The model under review builds one solid part; all positions refer to its coordinate system, in mm. A direction names the side the tool comes from. Round coordinates to 2 decimals unless told otherwise and drop trailing zeros. Order: outer loops, then holes, each group sorted by start corner. A loop starts at its lowest first (then second) coordinate and runs counter-clockwise, first axis right, second up.
1) Consider section A-A (y = 50). Give the boundary of the cut face in (x, z), then the cut area to 3 significant figures.
2) Consider section B-B (x = -3). Give the number of separate pieces and of enclosed holes in the cut face, then the cut area to 3 significant figures.
3) Clearance check with flat-ended pins moving along their axes: P1, Ø10.5, axis at x = -18, y = 14.5, coming from the -Z side; P2, Ø1.6, axis at x = -12.5, z = -1, coming from the +Y side; P3, Ø2.5, axis at x = -20, z = 3.5, coming from the +Y side; P4, Ø2.5, axis at x = 0, y = 59.563, coming from the -Z side. State where each tip first meets the part, or that it passes through.
4) Machinability: for faces 5 (the face through (-12, 0, -2)), 6 (the face through (12.29, 102.343, 3.073)), 7 (the face through (0, 0, 2)), which of the approach directions +Z, -Z, +X, -X, +Y, -Y give a long, thin tool a straight path to every point of the face, cutting with its end or side? Answer none if there is none.
5) Mouldability with a two-part tool opening along Y and no side actions: class faces 1 (the face through (-47.955, -39, 1)), 2 (the face through (-25.182, -23.28, -1.032)), 3 (the face through (17, 86.36, 2)), 4 (the face through (-0.05, 79.4, 2.44)) as pulls with the +Y half, pulls with the -Y half, needs draft (parallel to the pull), parting line crosses it, or undercut.
6) To check wall thickness, follow L1, parallel to Y at x = 1, z = 3.5; L2, parallel to Y at x = -21, z = -0.75; L3, parallel to Y at x = -8, z = 4.75. State the ranges of each line that lie inside material, in increasing order.
7) Consider section D-D (y = 93). Give the boundary of the cut face in (x, z), then the cut area to 3 significant figures.
from build123d import *

# Parameters (mm, degrees)
F1_DEPTH       = 4.953
F3_DEPTH       = 4.954
F5_DEPTH       = 109.983
F7_DEPTH       = 15.494
F8_W           = 74.6252
F8_H           = 44.45
F9_DEPTH       = 4.953
F9_DEPTH_BACK  = 3.175
F11_R          = 1.27
F17_DEPTH      = 3.176
F17_DEPTH_BACK = 4.954
F19_D          = 3.15
F20_R          = 3.302
F21_R          = 2.5393938838
F22_SIZE       = 2.286


# Not quite as in the source:
# - a feature names something its author has since deleted; it is built from what else it names


with BuildPart() as f1:
    # F0 (on Top) → F1 (new body)
    with BuildSketch(Plane.XY):
        Polygon((-26.67, 0), (26.67, 0), (26.67, 90.043), (16.9418, 109.982), (-16.9418, 109.982), (-26.67, 90.043), align=None)
    extrude(amount=F1_DEPTH)

    # F2 (on Top) → F3 (cut, through all)
    with BuildSketch(Plane.XY):
        with BuildLine():
            Line((-26.67, 28.0162), (-7.0612, 28.0162))
            ThreePointArc((-7.0612, 28.0162), (0.0508, 35.1282), (-7.0612, 42.2402))
            Line((-7.0612, 42.2402), (-26.67, 42.2402))
            Line((-26.67, 42.2402), (-26.67, 28.0162))
        make_face()
        with BuildLine():
            Line((26.67, 86.36), (7.0612, 86.36))
            ThreePointArc((7.0612, 86.36), (-0.0508, 79.248), (7.0612, 72.136))
            Line((7.0612, 72.136), (26.67, 72.136))
            Line((26.67, 72.136), (26.67, 86.36))
        make_face()
    extrude(amount=F3_DEPTH, mode=Mode.SUBTRACT)

    # F4 (on face) → F5 (cut, through all)
    with BuildSketch(Plane.XZ):
        with BuildLine():
            ThreePointArc((-11.0871, 0), (-12.3571, 1.27), (-13.6271, 0))
            Line((-13.6271, 0), (-11.0871, 0))
        make_face()
        with BuildLine():
            ThreePointArc((13.6271, 0), (12.3571, 1.27), (11.0871, 0))
            Line((11.0871, 0), (13.6271, 0))
        make_face()
    extrude(amount=-F5_DEPTH, mode=Mode.SUBTRACT)

    # F6 (on face) → F7 (cut)
    with BuildSketch(Plane(origin=(0, 109.982, 0), x_dir=(-1, 0, 0), z_dir=(0, 1, 0))):
        with BuildLine():
            ThreePointArc((-9.2837, 0), (-12.3571, 3.0734), (-15.4305, 0))
            Line((-15.4305, 0), (-9.2837, 0))
        make_face()
        with BuildLine():
            ThreePointArc((15.4305, 0), (12.3571, 3.0734), (9.2837, 0))
            Line((9.2837, 0), (15.4305, 0))
        make_face()
    extrude(amount=-F7_DEPTH, mode=Mode.SUBTRACT)

    # F8 (on Top) → F9 (join, two sides)
    with BuildSketch(Plane.XY) as f9_sk:
        with Locations((-10.6426, -22.225)):
            Rectangle(F8_W, F8_H)
    extrude(amount=F9_DEPTH)
    extrude(f9_sk.sketch, amount=-F9_DEPTH_BACK)

    # F12: sweep along a path in F10
    with BuildLine(Plane.XY) as f12_path:
        Line((-47.9552, -41.275), (-28.9179, -41.275))
        ThreePointArc((-28.9179, -41.275), (0.2679323935, -29.1858323935), (12.3571, 0))
    # F11 (on face) → F12 (sweep, cut)
    with BuildSketch(Plane(origin=(0, 0, 0), x_dir=(-1, 0, 0), z_dir=(0, 1, 0))):
        with Locations((-12.3571, 0)):
            Circle(F11_R)
    sweep(path=f12_path.line, mode=Mode.SUBTRACT)

    # F15: sweep along a path in F13
    with BuildLine(Plane.XY) as f15_path:
        ThreePointArc((-12.3571, 0), (-22.7835420926, -25.1716579074), (-47.9552, -35.5981))
    # F14 (on face) → F15 (sweep, cut)
    with BuildSketch(Plane(origin=(0, 0, 0), x_dir=(-1, 0, 0), z_dir=(0, 1, 0))):
        with BuildLine():
            ThreePointArc((11.0871, 0), (12.3571, -1.27), (13.6271, 0))
            ThreePointArc((13.6271, 0), (12.3571, 1.27), (11.0871, 0))
        make_face()
    sweep(path=f15_path.line, mode=Mode.SUBTRACT)

    # F16 (on Top) → F17 (cut, two sides)
    with BuildSketch(Plane.XY) as f17_sk:
        with BuildLine():
            Line((-28.9179, -44.45), (26.67, -44.45))
            Line((26.67, -44.45), (26.67, 0))
            Line((26.67, 0), (15.5321, 0))
            ThreePointArc((15.5321, 0), (2.5129964237, -31.4308964237), (-28.9179, -44.45))
        make_face()
        with BuildLine():
            ThreePointArc((-28.9179, -38.1), (-1.9771316368, -26.9407683632), (9.1821, 0))
            Line((9.1821, 0), (-9.1821, 0))
            ThreePointArc((-9.1821, 0), (-14.4660215428, -19.5404250178), (-28.8776213731, -33.7549889252))
            Line((-28.8776213731, -33.7549889252), (-28.9179, -38.1))
        make_face()
        with BuildLine():
            ThreePointArc((-47.9552, -32.4231), (-25.0286061229, -22.9265938771), (-15.5321, 0))
            Line((-15.5321, 0), (-47.9552, 0))
            Line((-47.9552, 0), (-47.9552, -32.4231))
        make_face()
    extrude(amount=-F17_DEPTH, mode=Mode.SUBTRACT)
    extrude(f17_sk.sketch, amount=F17_DEPTH_BACK, mode=Mode.SUBTRACT)

    # F19 (through all)
    with Locations(Plane.XY.offset(4.953)):
        with Locations((0, 99.1108), (0, 59.563), (0, 15.0622)):
            Hole(F19_D / 2)

    # F20
    f20_edges = [f1.edges().sort_by_distance(p)[0] for p in [
        (9.1821, 0, 2.4765),
        (-9.1821, 0, 2.4765),
        (15.5321, 0, 2.4765),
        (-15.5321, 0, 2.4765),
    ]]
    fillet(f20_edges, radius=F20_R)

    # F21
    f21_edges = [f1.edges().sort_by_distance(p)[0] for p in [
        (-28.877621, -33.754989, 0.889),
        (-28.9179, -38.1, 0.889),
    ]]
    fillet(f21_edges, radius=F21_R)

    # F22
    f22_edges = [f1.edges().sort_by_distance(p)[0] for p in [
        (-38.43655, -44.45, -3.175),
        (-14.121028, -18.936792, -3.175),
        (-28.561794, -33.963255, -3.175),
        (-28.892105, -35.317366, -3.175),
        (-28.092277, -37.319249, -3.175),
        (-1.022826, -25.951394, -3.175),
        (-25.028606, -22.926594, -3.175),
        (2.512996, -31.430896, -3.175),
    ]]
    chamfer(f22_edges, length=F22_SIZE)


solid = f1.part
Answer below:
1. outline: (-26.67, 0) - (-13.63, 0) arc R1.27 cw to (-11.09, 0) - (11.09, 0) arc R1.27 cw to (13.63, 0) - (26.67, 0) - (26.67, 4.95) - (-26.67, 4.95) - close
1. area: 259 mm2
2. separate pieces: 3
2. enclosed holes: 1
2. area: 540 mm2
3. P1: stops at z = 0
3. P2: stops at y = 0
3. P3: stops at y = 106.28
3. P4: passes through
4. face 5: -Z, +X, -X, +Y
4. face 6: -Z, +Y
4. face 7: +Z, -Z
5. face 1: needs draft
5. face 2: pulls with the +Y half
5. face 3: undercut
5. face 4: undercut
6. L1: y = -32.87 to -23.59, 0 to 13.85, 16.28 to 58.35, 60.78 to 75.53, 82.97 to 97.89, 100.33 to 109.98
6. L2: y = -43.74 to -41.55, -39.46 to -37.27, -27.87 to -24.79, -21.65 to -18.02
6. L3: y = -39.22 to -31.84, -0.67 to 28.02, 42.24 to 109.98
7. outline: (-25.23, 0) - (-13.63, 0) arc R1.27 cw to (-11.09, 0) - (11.09, 0) arc R1.27 cw to (13.63, 0) - (25.23, 0) - (25.23, 4.95) - (-25.23, 4.95) - close
7. area: 245 mm2
